Can you work these out from the model? Positions are in its coordinate system, mm. Face numbers are marked on the shaded views. A direction names the side the tool comes from. Coordinates: 2 decimals unless noted, no trailing zeros. Loops run counter-clockwise (first coordinate to the right, second up) from the corner with the lowest first, then second, coordinate; pieces in that order, holes last. Notation, with made-up numbers: (15, 41.25) -> (71, 41.25) arc R17 ccw to (71, 50.25) -> close; hole circle Ø7 at (-30.5, -11.75). An arc over 180 degrees is marked (long way). Use one line per item in the form item = value. Start each with the question number.
(1) Imagine slicing it at A-A (x = -6). List the corners of the cut face in (y, z) for me, plus the area to 3 significant figures.
(2) I need wall thicknesses on line 1 (Z direction, x = 5, y = 0); line 2 (X direction, y = -10.25, z = -0.25); line 3 (Y direction, x = -5, z = 0). Which ranges of each line are inside material? Lowest first, please. Write a range as [from, to].
(3) I'm going to push flat-ended pins straight in: pin 1 (4 mm diameter, centred on x = -18, z = 7, fed in from -Y); pin 2 (10 mm diameter, centred on x = 16.5, y = -10, fed in from +Z); pin 3 (5 mm diameter, centred on x = -17.5, y = 3.5, fed in from +Z); pin 4 (10 mm diameter, centred on y = -10, z = -8, fed in from -X). Where does each tip first touch, or does it pass through?
(4) Thinking about a two-plate mould opening in X: for the marked faces 5, 6 and 7, which applies, released by +X, released by -X, zero draft, split by the parting line, or undercut?
(5) On a 3-axis mill with a long thin cutter (end or side, diameter ignored), from which of +Z, -Z, +X, -X, +Y, -Y can I reach the whole of each face in a straight line? I mean the marked faces 1, 2, 3 and 4. Say none if no direction works.
(6) Imagine slicing it at B-B (x = 16.5). List the corners of the cut face in (y, z) for me.
Autodesk Inventor part; units mm, degrees
ref_plane "YZ Plane" through (0, 0, 0) normal (1, 0, 0) x (0, 1, 0)
ref_plane "XZ Plane" through (0, 0, 0) normal (0, 1, 0) x (-1, 0, 0)
ref_plane "XY Plane" through (0, 0, 0) normal (0, 0, 1) x (1, 0, 0)
sketch "Эскиз1" plane through (0, 0, 0) normal (0, 0, 1) x (1, 0, 0)
  line L0 (-24, 0) -> (24, 0)
  line L1 (0, -5.5) -> (-23.2, -5.5)
  line L2 (-24, -6.3) -> (-24, -10.4)
  line L3 (0, -5.5) -> (0, -6)
  line L4 (0, -6) -> (24, -6)
  line L5 (-23.2, -5.5) -> (-24, -6.3)
  line L6 (-22.4, -12) -> (-2.2, -12)
  line L7 (-22.4, -12) -> (-24, -10.4)
  line L8 (-1.4, -11.2) -> (-1.4, -11)
  line L9 (-1.4, -11) -> (1.6, -11)
  line L10 (-2.2, -12) -> (-1.4, -11.2)
  line L11 (1.6, -11) -> (1.6, -13.5)
  line L12 (2.1, -14) -> (7.1, -14)
  line L13 (7.6, -13.5) -> (7.6, -9.5)
  line L14 (7.6, -9.5) -> (12.6, -9.5)
  line L15 (2.1, -14) -> (1.6, -13.5)
  line L16 (7.1, -14) -> (7.6, -13.5)
  line L17 (12.6, -9.5) -> (12.6, -11)
  line L18 (12.6, -11) -> (21.6, -11)
  line L19 (21.6, -11) -> (21.6, -9.5)
  line L20 (24, -6) -> (23, -6.2309)
  line L21 (23, -6.2309) -> (23, -9.5)
  line L22 (23, -9.5) -> (21.6, -9.5)
  point P0 (0, 0)
  point P1 (0, 0)
  point P2 (-24, -5.5)
  point P3 (-24, -12)
  point P4 (-1.4, -12)
  point P5 (1.6, -14)
  point P6 (7.6, -14)
  dimension "d0" = 48
  dimension "d24" = 12
  dimension "d25" = 11
  dimension "d26" = 24
  dimension "d27" = 0.8
  dimension "d28" = 45
  dimension "d29" = 24
  dimension "d30" = 1.6
  dimension "d31" = 45
  dimension "d32" = 22
  dimension "d33" = 0.8
  dimension "d34" = 45
  dimension "d35" = 3
  dimension "d36" = 24
  dimension "d37" = 0.5
  dimension "d38" = 45
  dimension "d39" = 0.5
  dimension "d40" = 45
  dimension "d41" = 19
  dimension "d42" = 6
  dimension "d43" = 5
  dimension "d44" = 22
  dimension "d47" = 13
  dimension "d49" = 14
  dimension "d50" = 19
  dimension "d51" = 1
  dimension "d52" = 28
revolve "Вращение1" add sketch "Эскиз1" angle 360 about axis through (-24, 0, 0) along (1, 0, 0)
sketch "Эскиз2" plane through (0, 0, 0) normal (0, 1, 0) x (-1, 0, 0)
  line L0 (-1.6, -13.5) -> (-1.6, 13.5)
  line L1 (-7.1, 14) -> (-2.1, 14)
  line L2 (-7.6, 13.5) -> (-7.1, 14)
  line L3 (-7.6, -13.5) -> (-7.6, 13.5)
  line L4 (-2.1, 14) -> (-1.6, 13.5)
  line L5 (-3.6, 14) -> (-3.6, 12)
  line L6 (-3.6, 12) -> (-7.6, 12)
  line L7 (2.2, 12) -> (22.4, 12)
  point P0 (0, 0)
  dimension "d54" = 2
extrude "Выдавливание1" cut sketch "Эскиз2" along normal through all both and the other way through all
fillet "Сопряжение1" radius 0.3 1 edges at (3.6, 0, 12)
thread "Резьба1"
equation "\"d40\" = d38"
properties part number "411. Штуцер гибкого вала"
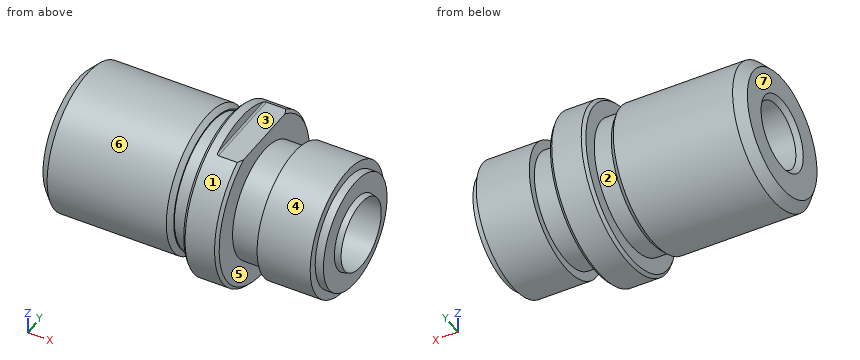
Worked out:
q1.outline = circle Ø24 at (0, 0); hole circle Ø11 at (0, 0)
q1.area = 357 mm2
q2.line_1 = [-14, -6], [6, 12]
q2.line_2 = [-24, 7.6], [12.6, 21.6]
q2.line_3 = [-12, -5.5], [5.5, 12]
q3.pin_1 = -10.91
q3.pin_2 = 9.8
q3.pin_3 = 11.96
q3.pin_4 = -24
q4.face_5 = undercut
q4.face_6 = zero draft
q4.face_7 = released by -X
q5.face_1 = +X, -X
q5.face_2 = none
q5.face_3 = +Z, +X, +Y, -Y
q5.face_4 = +X
q6.outline = circle Ø22 at (0, 0); hole circle Ø12 at (0, 0)
